Can you work these out from the model? Positions are in its coordinate system, mm. Round coordinates to 2 decimals unless told otherwise and drop trailing zeros. Write each loop counter-clockwise with the first axis right and the second up, starting at its lowest first coordinate (ties: lowest second). Pieces come first, ordered by that corner, then holes.
Q1. I'm going to push flat-ended pins straight in: pin 1 Ø1.5 at (x, y) = (-51.5, -1) entering from +Z; pin 2 Ø0.6 at (y, z) = (0, 3.5) entering from -X. Where does each tip first touch, or does it pass through?
Q2. If we section it at B-B (y = 1.4): Please give me the cut outline in (x, z), plus the area to 3 significant figures.
Q3. If we section it at A-A (z = 3.9): Please give me the cut outline in (x, y).
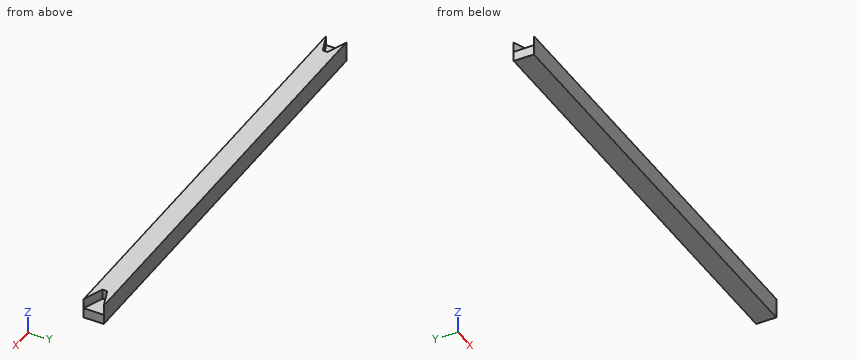
from build123d import *

# Parameters (mm, degrees)
SKETCH_W     = 110
SKETCH_H     = 5
PAD_DEPTH    = 2.5
PAD001_DEPTH = 2.5


with BuildPart() as part:
    # Sketch → Pad (new body)
    with BuildSketch(Plane.XY):
        Rectangle(SKETCH_W, SKETCH_H)
    extrude(amount=PAD_DEPTH)

    # Sketch001 → Pad001 (new body)
    with BuildSketch(Plane.XY.offset(2.5)):
        Polygon((-55, 2.5), (55, 2.5), (50, 0.6), (50, -0.6), (55, -2.5), (-55, -2.5), (-50, -0.6), (-50, 0.6), align=None)
    extrude(amount=PAD001_DEPTH)


solid = part.part
A:
1. pin 1: stops at z = 5
1. pin 2: stops at x = -50
2. outline: (-55, 0) - (55, 0) - (55, 2.5) - (52.11, 2.5) - (52.11, 5) - (-52.11, 5) - (-52.11, 2.5) - (-55, 2.5) - close
2. area: 536 mm2
3. outline: (-55, -2.5) - (55, -2.5) - (50, -0.6) - (50, 0.6) - (55, 2.5) - (-55, 2.5) - (-50, 0.6) - (-50, -0.6) - close
